from build123d import *

# Parameters (mm, degrees)
SKETCH1_W                                           = 150
SKETCH1_H                                           = 150
BOSS_EXTRUDE1_DEPTH                                 = 20
M10_TAPPED_HOLE1_D                                  = 8.5
CBORE_FOR_M5_HEX_SOCKET_HEAD_CAP_SCREW1_D           = 5.5
CBORE_FOR_M5_HEX_SOCKET_HEAD_CAP_SCREW1_CBORE_D     = 10
CBORE_FOR_M5_HEX_SOCKET_HEAD_CAP_SCREW1_CBORE_DEPTH = 5.5
F_5_5_5_5_DIAMETER_HOLE1_D                          = 5.5
SKETCH6_R                                           = 50
CUT_EXTRUDE1_DEPTH                                  = 5
FILLET1_R                                           = 1
CHAMFER2_SIZE                                       = 1
CUT_EXTRUDE2_DEPTH                                  = 10


with BuildPart() as part:
    # Sketch1 → Boss-Extrude1 (new body)
    with BuildSketch(Plane.XY):
        Rectangle(SKETCH1_W, SKETCH1_H)
    extrude(amount=BOSS_EXTRUDE1_DEPTH)

    # M10 Tapped Hole1 (through all)
    with Locations(Plane.XY.offset(20)):
        with Locations((0, 0)):
            Hole(M10_TAPPED_HOLE1_D / 2)

    # CBORE for M5 Hex Socket Head Cap Screw1 (through all)
    with Locations(Plane.XY.offset(20)):
        with Locations((-65, 65), (-45, 65), (-65, 45), (65, -45), (65, -65), (45, -65), (45, 65), (65, 65), (65, 45), (45, -45), (-45, 45), (45, 45)):
            CounterBoreHole(CBORE_FOR_M5_HEX_SOCKET_HEAD_CAP_SCREW1_D / 2, CBORE_FOR_M5_HEX_SOCKET_HEAD_CAP_SCREW1_CBORE_D / 2, CBORE_FOR_M5_HEX_SOCKET_HEAD_CAP_SCREW1_CBORE_DEPTH)

    # Ø5.5 (5.5) Diameter Hole1 (through all)
    with Locations(Plane.XY.offset(20)):
        with Locations((-65, -45), (-45, -45), (-45, -65), (-65, -65)):
            Hole(F_5_5_5_5_DIAMETER_HOLE1_D / 2)

    # Sketch6 → Cut-Extrude1 (cut)
    with BuildSketch(Plane.XY.offset(20)):
        Circle(SKETCH6_R)
    extrude(amount=-CUT_EXTRUDE1_DEPTH, mode=Mode.SUBTRACT)

    # Fillet1
    fillet1_edges = [part.edges().sort_by_distance(p)[0] for p in [
        (-50, 0, 15),
    ]]
    fillet(fillet1_edges, radius=FILLET1_R)

    # Chamfer2
    chamfer2_edges = [part.edges().sort_by_distance(p)[0] for p in [
        (-50, 0, 20),
    ]]
    chamfer(chamfer2_edges, length=CHAMFER2_SIZE)

    # Sketch7 → Cut-Extrude2 (cut)
    with BuildSketch(Plane.XY.offset(20)):
        with BuildLine():
            Line((-75, -75), (-34.5, -75))
            Line((-34.5, -75), (-34.5, -45))
            ThreePointArc((-34.5, -45), (-37.575378798, -37.575378798), (-45, -34.5))
            Line((-45, -34.5), (-75, -34.5))
            Line((-75, -34.5), (-75, -75))
        make_face()
    extrude(amount=-CUT_EXTRUDE2_DEPTH, mode=Mode.SUBTRACT)


solid = part.part
CAD build for the part. Positions are in the model's coordinates, mm. A direction names the side the tool comes from. Coordinates: 2 decimals unless noted, no trailing zeros. Loops run counter-clockwise (first coordinate to the right, second up) from the corner with the lowest first, then second, coordinate; pieces in that order, holes last. Notation, with made-up numbers: (62.5, 69.25) - (72.5, 69.25) arc R17 cw to (72.5, 79.25) - close; hole circle Ø8 at (-13.5, -29). An arc over 180 degrees is marked (long way). Use one line per item in the form item = value. Start each with the question number.
1) Drill centre lines: L1, parallel to Y at x = 45, z = 3.75; L2, parallel to Y at x = -65, z = 16.9; L3, parallel to Y at x = 65, z = 17.3. Where is each one in solid material? Low to high. Write a range as from..to.
2) Tool access for faces 4 (the face through (47.027, -43.141, 7.148)), 5 (the face through (67.2, -47.2, 14.5)): list every direction of +Z, -Z, +X, -X, +Y, -Y with a clear straight run to the whole face (end or side of a thin tool).
3) Band-saw the part on B-B (x = 0). Give the cut face in (y, z).
4) Band-saw the part on A-A (y = -65). State how many separate pieces and enclosed holes the cut face has, and give its area (3 significant figures).
5) Two-plate mould, pull along X, no slides. Class faces 1 (the face through (-55, -54, 10)), 2 (the face through (75, -1, 10)), 3 (the face through (68, 69, 17)): +X half, -X half, draft (parallel to the pull), parting line (faces both ways), or undercut.
6) Flat gauge pins, fed straight in: pin 1 (8 mm diameter, centred on x = -45, y = 65, fed in from +Z); pin 2 (7 mm diameter, centred on x = -65, y = -65, fed in from +Z); pin 3 (3 mm diameter, centred on x = -54.5, z = 15.5, fed in from -Y). Where does each tip first touch, or does it go through?
Check values:
q1.L1 = -75..-67.75, -62.25..-47.75, -42.25..42.25, 47.75..62.25, 67.75..75
q1.L2 = -34.5..40, 50..60, 70..75
q1.L3 = -75..-70, -60..-50, -40..40, 50..60, 70..75
q2.face_4 = +Z, -Z
q2.face_5 = +Z
q3.outline = (-75, 0) - (-4.25, 0) - (-4.25, 15) - (-49, 15) arc R1 cw to (-50, 16) - (-50, 19) - (-51, 20) - (-75, 20) - close; (4.25, 0) - (75, 0) - (75, 20) - (51, 20) - (50, 19) - (50, 16) arc R1 cw to (49, 15) - (4.25, 15) - close
q4.separate_pieces = 5
q4.enclosed_holes = 0
q4.area = 2,220 mm2
q5.face_1 = draft
q5.face_2 = +X half
q5.face_3 = undercut
q6.pin_1 = 14.5
q6.pin_2 = 10
q6.pin_3 = -34.5
